from build123d import *

# Parameters (mm, degrees)
SKETCH1_W           = 5.7404
SKETCH1_H           = 7.112
BOSS_EXTRUDE1_DEPTH = 10.414
CUT_EXTRUDE1_START  = -2.54
SKETCH3_W           = 12.1412
SKETCH3_H           = 7.62
CUT_EXTRUDE1_DEPTH  = 19.5072
SKETCH4_W           = 10.922
SKETCH4_H           = 7.62
CUT_EXTRUDE2_DEPTH  = 73.133620947
CUT_EXTRUDE3_DEPTH  = 48.257817764
SKETCH6_R           = 3.175
BOSS_EXTRUDE2_DEPTH = 4.8768


with BuildPart() as part:
    # Sketch1 → Boss-Extrude1 (new body)
    with BuildSketch(Plane(origin=(0, 0, 0), x_dir=(1, 0, 0), z_dir=(0, 1, 0))):
        Polygon((-41.148, -10.16), (-27.559, -10.16), (-27.559, 0), (27.559, 0), (27.559, -10.16), (41.148, -10.16), (41.148, -1.524), (29.0449, 13.1572), (-29.0449, 13.1572), (-41.148, -1.524), align=None)
        with Locations((7.62, 5.9055)):
            Rectangle(SKETCH1_W, SKETCH1_H, mode=Mode.SUBTRACT)
        with Locations((0, 5.9055)):
            Rectangle(SKETCH1_W, SKETCH1_H, mode=Mode.SUBTRACT)
        with Locations((15.24, 5.9055)):
            Rectangle(SKETCH1_W, SKETCH1_H, mode=Mode.SUBTRACT)
        with Locations((22.86, 5.9055)):
            Rectangle(SKETCH1_W, SKETCH1_H, mode=Mode.SUBTRACT)
        with Locations((-7.62, 5.9055)):
            Rectangle(SKETCH1_W, SKETCH1_H, mode=Mode.SUBTRACT)
        with Locations((-15.24, 5.9055)):
            Rectangle(SKETCH1_W, SKETCH1_H, mode=Mode.SUBTRACT)
        with Locations((-22.86, 5.9055)):
            Rectangle(SKETCH1_W, SKETCH1_H, mode=Mode.SUBTRACT)
    extrude(amount=BOSS_EXTRUDE1_DEPTH)

    # Sketch3 → Cut-Extrude1 (cut)
    with BuildSketch(Plane.XY.offset(10.16).offset(CUT_EXTRUDE1_START)):
        with Locations((35.0774, 5.207)):
            Rectangle(SKETCH3_W, SKETCH3_H)
    cut_extrude1 = extrude(amount=-CUT_EXTRUDE1_DEPTH, mode=Mode.SUBTRACT)

    # Sketch4 → Cut-Extrude2 (cut, through all)
    with BuildSketch(Plane(origin=(29.0068, 0, 0), x_dir=(0, 0, -1), z_dir=(1, 0, 0))):
        with Locations((6.4262, 5.207)):
            Rectangle(SKETCH4_W, SKETCH4_H)
    extrude(amount=-CUT_EXTRUDE2_DEPTH, mode=Mode.SUBTRACT)

    # Sketch5 → Cut-Extrude3 (cut, through all)
    with BuildSketch(Plane(origin=(0, 0, 7.62), x_dir=(-1, 0, 0), z_dir=(0, 0, -1))):
        with BuildLine():
            Line((-34.4043, 3.0607), (-36.9697, 3.0607))
            ThreePointArc((-36.9697, 3.0607), (-39.116, 5.207), (-36.9697, 7.3533))
            Line((-36.9697, 7.3533), (-34.4043, 7.3533))
            ThreePointArc((-34.4043, 7.3533), (-32.258, 5.207), (-34.4043, 3.0607))
        make_face()
    cut_extrude3 = extrude(amount=-CUT_EXTRUDE3_DEPTH, mode=Mode.SUBTRACT)

    # Mirror1: Cut-Extrude1, Cut-Extrude3 across plane
    add(cut_extrude1.mirror(Plane(origin=(0, 0, 0), x_dir=(0, 0, 1), z_dir=(1, 0, 0))), mode=Mode.SUBTRACT)
    add(cut_extrude3.mirror(Plane(origin=(0, 0, 0), x_dir=(0, 0, 1), z_dir=(1, 0, 0))), mode=Mode.SUBTRACT)

    # Sketch6 → Boss-Extrude2 (add)
    with BuildSketch(Plane(origin=(0, 0, -13.1572), x_dir=(-1, 0, 0), z_dir=(0, 0, -1))):
        with BuildLine():
            ThreePointArc((-3.81, 3.602218207), (0, 0.92820964), (3.81, 3.602218207))
            ThreePointArc((3.81, 3.602218207), (7.62, 0.92820964), (11.43, 3.602218207))
            ThreePointArc((11.43, 3.602218207), (15.24, 0.92820964), (19.05, 3.602218207))
            ThreePointArc((19.05, 3.602218207), (26.9113, 4.97950964), (19.05, 6.356801072))
            ThreePointArc((19.05, 6.356801072), (15.24, 9.03080964), (11.43, 6.356801072))
            ThreePointArc((11.43, 6.356801072), (7.62, 9.03080964), (3.81, 6.356801072))
            ThreePointArc((3.81, 6.356801072), (0, 9.03080964), (-3.81, 6.356801072))
            ThreePointArc((-3.81, 6.356801072), (-7.62, 9.03080964), (-11.43, 6.356801072))
            ThreePointArc((-11.43, 6.356801072), (-15.24, 9.03080964), (-19.05, 6.356801072))
            ThreePointArc((-19.05, 6.356801072), (-26.9113, 4.97950964), (-19.05, 3.602218207))
            ThreePointArc((-19.05, 3.602218207), (-15.24, 0.92820964), (-11.43, 3.602218207))
            ThreePointArc((-11.43, 3.602218207), (-7.62, 0.92820964), (-3.81, 3.602218207))
        make_face()
        with Locations((0, 4.97950964)):
            Circle(SKETCH6_R, mode=Mode.SUBTRACT)
        with Locations((7.62, 4.97950964)):
            Circle(SKETCH6_R, mode=Mode.SUBTRACT)
        with Locations((15.24, 4.97950964)):
            Circle(SKETCH6_R, mode=Mode.SUBTRACT)
        with Locations((22.86, 4.97950964)):
            Circle(SKETCH6_R, mode=Mode.SUBTRACT)
        with Locations((-7.62, 4.97950964)):
            Circle(SKETCH6_R, mode=Mode.SUBTRACT)
        with Locations((-15.24, 4.97950964)):
            Circle(SKETCH6_R, mode=Mode.SUBTRACT)
        with Locations((-22.86, 4.97950964)):
            Circle(SKETCH6_R, mode=Mode.SUBTRACT)
    extrude(amount=BOSS_EXTRUDE2_DEPTH)


solid = part.part
Can you work these out from the model? Positions are in its coordinate system, mm. A direction names the side the tool comes from. Give positions to 0.01 mm unless a question says otherwise; leave off trailing zeros. Loops run counter-clockwise (first coordinate to the right, second up) from the corner with the lowest first, then second, coordinate; pieces in that order, holes last. Notation, with made-up numbers: (3.5, 33.25) -> (34.5, 33.25) arc R26 ccw to (34.5, 64.25) -> close; hole circle Ø1 at (58, -29.5). An arc over 180 degrees is marked (long way). Return JSON: item names as keys, results as strings.
Q1. I need wall thicknesses on probe 1 along Y at (x, z) = (-23, -1.5); probe 2 along X at (y, z) = (3, 3.25); probe 3 along Y at (x, z) = (-22.86, -15.65). Which ranges of each line are inside material? Lowest first, please.
Checks:
{"probe 1": "y = 0 to 1.4, 9.02 to 10.41", "probe 2": "x = -29.01 to -27.56, 27.56 to 29.01", "probe 3": "y = 0.93 to 1.8, 8.15 to 9.03"}
Q2. I want a section at A-A, the plane z = 5.5. List the corners of the cut face in (x, y) for me, then the cut area to 3 significant figures.
Checks:
{"outline": "(-41.15, 0) -> (-27.56, 0) -> (-27.56, 10.41) -> (-41.15, 10.41) -> (-41.15, 9.02) -> (-29.01, 9.02) -> (-29.01, 1.4) -> (-41.15, 1.4) -> close; (27.56, 0) -> (41.15, 0) -> (41.15, 1.4) -> (29.01, 1.4) -> (29.01, 9.02) -> (41.15, 9.02) -> (41.15, 10.41) -> (27.56, 10.41) -> close", "area": "98.0 mm2"}
Q3. I want a section at D-D, the plane z = -5.75. Count the separate pieces of the cut face and the enclosed holes in it, then the cut area to 3 significant figures.
Checks:
{"separate pieces": "16", "enclosed holes": "0", "area": "84.2 mm2"}
Q4. We'd pull the mould along Z, two halves only. Please class faces 1 (the face through (12.37, 1, -6)), 2 (the face through (-8, 5, -13.157)), 3 (the face through (-10.65, 5.93, -15.56)): released by +Z, released by -Z, zero draft, split by the parting line, or undercut.
Checks:
{"face 1": "undercut", "face 2": "released by -Z", "face 3": "zero draft"}
Q5. I want a section at C-C, the plane x = 15.24. List the corners of the cut face in (y, z) for me.
Checks:
{"outline": "(0, -13.16) -> (0.93, -13.16) -> (0.93, -18.03) -> (1.8, -18.03) -> (1.8, -13.16) -> (8.15, -13.16) -> (8.15, -18.03) -> (9.03, -18.03) -> (9.03, -13.16) -> (10.41, -13.16) -> (10.41, -9.46) -> (9.02, -9.46) -> (9.02, -11.89) -> (1.4, -11.89) -> (1.4, -9.46) -> (0, -9.46) -> close; (0, -2.35) -> (1.4, -2.35) -> (1.4, -0.97) -> (9.02, -0.97) -> (9.02, -2.35) -> (10.41, -2.35) -> (10.41, 0) -> (0, 0) -> close"}
Q6. I want a section at B-B, the plane x = -33.5. List the corners of the cut face in (y, z) for me, then the cut area to 3 significant figures.
Checks:
{"outline": "(0, -7.75) -> (1.4, -7.75) -> (1.4, 7.62) -> (3.26, 7.62) -> (3.26, 10.16) -> (0, 10.16) -> close; (7.15, 7.62) -> (9.02, 7.62) -> (9.02, -7.75) -> (10.41, -7.75) -> (10.41, 10.16) -> (7.15, 10.16) -> close", "area": "59.5 mm2"}
Q7. On a 3-axis mill with a long thin cutter (end or side, diameter ignored), from which of +Z, -Z, +X, -X, +Y, -Y can I reach the whole of each face in a straight line? I mean faces 4 (the face through (36, 7.353, 9)), 5 (the face through (-15, 10, -2.35)). Say none if no direction works.
Checks:
{"face 4": "+Z, -Z", "face 5": "+Y, -Y"}
Q8. For pin 1 Ø1 at (x, y) = (13, 8) entering from +Z; pin 2 Ø1.9 at (x, y) = (7.5, 4.5) entering from -Z; pin 3 Ø2.5 at (x, y) = (34.5, 4) entering from -Z, each with a flat end and sliding along its axis, tell me the tip position at first contact or that it passes through.
Checks:
{"pin 1": "stops at z = 0", "pin 2": "stops at z = -13.16", "pin 3": "stops at z = 7.62"}
